Here's how the part is built. I have some questions about the finished solid (model axes, mm). Face numbers are marked on the shaded views. A direction names the side the tool comes from. Round coordinates to 2 decimals unless told otherwise and drop trailing zeros. Write each loop counter-clockwise with the first axis right and the second up, starting at its lowest first coordinate (ties: lowest second). Pieces come first, ordered by that corner, then holes. Notation, with made-up numbers: (-1, -21) - (22, -21) arc R37 cw to (22, 15) - close; hole circle Ø8 at (2, -17). An arc over 180 degrees is marked (long way). Use one line per item in the form item = value. Start each with the question number.
1. Will these pins go through, and if not, where does the flat tip stop? pin 1 (2 mm diameter, centred on x = 65, y = -36, fed in from +Z); pin 2 (10 mm diameter, centred on x = 101.5, z = -59.5, fed in from +Y); pin 3 (1 mm diameter, centred on y = -36, z = -41.5, fed in from +X); pin 4 (3 mm diameter, centred on x = 8.982, z = -11.956, fed in from +Y).
2. I want a section at A-A, the plane x = 96.5. List the corners of the cut face in (y, z) for me, plus the area to 3 significant figures.
3. I want a section at B-B, the plane z = -51.5. List the corners of the cut face in (x, y) for me.
4. Which directions (+Z, -Z, +X, -X, +Y, -Y) give clear straight access to the entire face, cutting with the end or side of a thin tool? Please do the marked faces 1 and 2.
5. We'd pull the mould along Z, two halves only. Please class the marked faces 3 and 4: +Z half, -Z half, draft (parallel to the pull), parting line (faces both ways), or undercut.
6. If I drill on line 1 along Z through (x, y) = (30.5, -38); line 2 along Z through (x, y) = (94.5, -36.25); line 3 along Z through (x, y) = (9, -37.75), over which ranges is the centre line in solid material (lowest first)?
```python
from build123d import *

# Parameters (mm, degrees)
P_IDAT_VYSUNUT_M1_DEPTH      = 2.5
SKICA2_W                     = 43.3
SKICA2_H                     = 10.4
SKICA2_W_2                   = 10.4
SKICA2_H_2                   = 43.3
ODEBRAT_VYSUNUT_M1_DEPTH     = 139.549375892
SKICA6_W                     = 120
SKICA6_H                     = 6.95
P_IDAT_VYSUNUT_M3_DEPTH      = 2
SKICA7_W                     = 5.554617132
SKICA7_H                     = 57.2
SKICA7_W_2                   = 6.443355873
P_IDAT_VYSUNUT_M4_DEPTH      = 2
SKICA3_R                     = 3
P_IDAT_VYSUNUT_M2_DEPTH      = 4
F_2_2_2_2_PR_M_R_D_RY1_D     = 2.2
F_2_2_2_2_PR_M_R_D_RY1_DEPTH = 10
ZAOBLIT1_R                   = 1
SKICA8_W                     = 2.8
SKICA8_H                     = 57.2
ODEBRAT_VYSUNUT_M3_DEPTH     = 139.58455752
F_3_5_3_5_PR_M_R_D_RY1_D     = 3.5
F_3_5_3_5_PR_M_R_D_RY1_DEPTH = 10


with BuildPart() as part:
    # Skica1 → Přidat vysunutím1 (new body)
    with BuildSketch(Plane.XZ.offset(39.4)):
        with BuildLine():
            Line((-4.318, -71.206), (-4.318, -3.206))
            ThreePointArc((-4.318, -3.206), (-2.853533906, 0.329533906), (0.682, 1.794))
            Line((0.682, 1.794), (110.682, 1.794))
            ThreePointArc((110.682, 1.794), (114.217533906, 0.329533906), (115.682, -3.206))
            Line((115.682, -3.206), (115.682, -71.206))
            ThreePointArc((115.682, -71.206), (114.217533906, -74.741533906), (110.682, -76.206))
            Line((110.682, -76.206), (0.682, -76.206))
            ThreePointArc((0.682, -76.206), (-2.853533906, -74.741533906), (-4.318, -71.206))
        make_face()
    extrude(amount=-P_IDAT_VYSUNUT_M1_DEPTH)

    # Skica2 → Odebrat vysunutím1 (cut, through all)
    with BuildSketch(Plane(origin=(0, -36.9, 0), x_dir=(1, 0, 0), z_dir=(0, 1, 0))):
        with Locations((55.682, 3.406)):
            Rectangle(SKICA2_W, SKICA2_H)
        with Locations((0.882, 37.206)):
            Rectangle(SKICA2_W_2, SKICA2_H_2)
        with Locations((55.682, 71.006)):
            Rectangle(SKICA2_W, SKICA2_H)
    extrude(amount=-ODEBRAT_VYSUNUT_M1_DEPTH, mode=Mode.SUBTRACT)

    # Skica6 → Přidat vysunutím3 (add)
    with BuildSketch(Plane(origin=(0, -36.9, 0), x_dir=(1, 0, 0), z_dir=(0, 1, 0))):
        with Locations((55.682, 12.081)):
            Rectangle(SKICA6_W, SKICA6_H)
        with Locations((55.682, 62.331)):
            Rectangle(SKICA6_W, SKICA6_H)
    extrude(amount=P_IDAT_VYSUNUT_M3_DEPTH)

    # Skica7 → Přidat vysunutím4 (add)
    with BuildSketch(Plane(origin=(0, -36.9, 0), x_dir=(1, 0, 0), z_dir=(0, 1, 0))):
        with Locations((105.633212162, 37.206)):
            Rectangle(SKICA7_W, SKICA7_H)
        with Locations((11.204720922, 37.206)):
            Rectangle(SKICA7_W_2, SKICA7_H)
    extrude(amount=P_IDAT_VYSUNUT_M4_DEPTH)

    # Skica3 → Přidat vysunutím2 (add)
    with BuildSketch(Plane(origin=(0, -36.9, 0), x_dir=(1, 0, 0), z_dir=(0, 1, 0))):
        with Locations(Location((30.432, 11.506, 0), (0, 0, 255.164888418))):
            Circle(SKICA3_R)
        with Locations(Location((8.982, 11.956, 0), (0, 0, 270))):
            Circle(SKICA3_R)
        with Locations(Location((8.982, 62.456, 0), (0, 0, 270))):
            Circle(SKICA3_R)
        with Locations(Location((30.432, 62.906, 0), (0, 0, 104.835111582))):
            Circle(SKICA3_R)
        with Locations(Location((80.932, 62.906, 0), (0, 0, 75.164888418))):
            Circle(SKICA3_R)
        with Locations(Location((80.932, 11.506, 0), (0, 0, 284.835111582))):
            Circle(SKICA3_R)
    extrude(amount=P_IDAT_VYSUNUT_M2_DEPTH)

    # Ø2.2 (2.2) průměr díry1
    with Locations(Plane(origin=(0, -39.4, 0), x_dir=(-1, 0, 0), z_dir=(0, -1, 0))):
        with Locations((-8.982, 62.456), (-30.432, 62.906), (-80.932, 62.906), (-80.932, 11.506), (-30.432, 11.506), (-8.982, 11.956)):
            Hole(F_2_2_2_2_PR_M_R_D_RY1_D / 2, depth=F_2_2_2_2_PR_M_R_D_RY1_DEPTH)

    # Zaoblit1
    zaoblit1_edges = [part.edges().sort_by_distance(p)[0] for p in [
        (80.932, -36.9, -8.506),
        (80.932, -36.9, -65.906),
        (30.432, -36.9, -65.906),
    ]]
    fillet(zaoblit1_edges, radius=ZAOBLIT1_R)

    # Skica8 → Odebrat vysunutím3 (cut, through all)
    with BuildSketch(Plane(origin=(0, -36.9, 0), x_dir=(1, 0, 0), z_dir=(0, 1, 0))):
        with Locations((-2.918, 37.206)):
            Rectangle(SKICA8_W, SKICA8_H)
        with Locations((114.282, 37.206)):
            Rectangle(SKICA8_W, SKICA8_H)
    extrude(amount=ODEBRAT_VYSUNUT_M3_DEPTH, mode=Mode.SUBTRACT)

    # Ø3.5 (3.5) průměr díry1
    with Locations(Plane(origin=(0, -39.4, 0), x_dir=(-1, 0, 0), z_dir=(0, -1, 0))):
        with Locations((0, 2.696455625), (-0.682, 71.206), (-110.682, 71.206), (-110.682, 3.206)):
            Hole(F_3_5_3_5_PR_M_R_D_RY1_D / 2, depth=F_3_5_3_5_PR_M_R_D_RY1_DEPTH)


solid = part.part
```
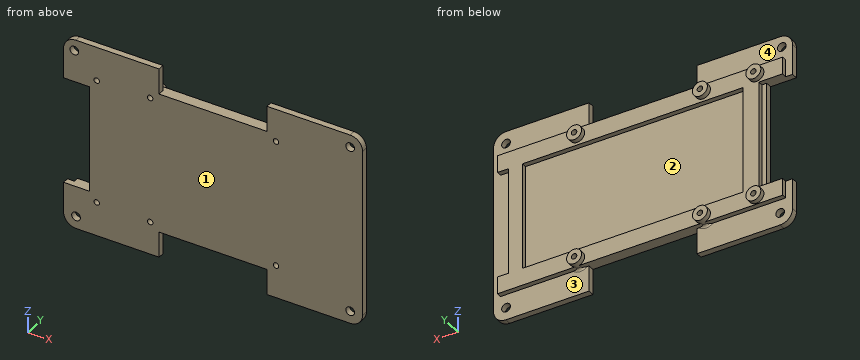
Model answer:
q1.pin_1 = -8.61
q1.pin_2 = -34.9
q1.pin_3 = 108.41
q1.pin_4 = -32.9
q2.outline = (-39.4, -76.21) - (-36.9, -76.21) - (-36.9, -65.81) - (-34.9, -65.81) - (-34.9, -58.86) - (-36.9, -58.86) - (-36.9, -15.56) - (-34.9, -15.56) - (-34.9, -8.61) - (-36.9, -8.61) - (-36.9, 1.79) - (-39.4, 1.79) - close
q2.area = 223 mm2
q3.outline = (6.08, -39.4) - (115.68, -39.4) - (115.68, -36.9) - (108.41, -36.9) - (108.41, -34.9) - (102.86, -34.9) - (102.86, -36.9) - (14.43, -36.9) - (14.43, -34.9) - (7.98, -34.9) - (7.98, -36.9) - (6.08, -36.9) - close
q4.face_1 = +Z, -Z, +X, -X, -Y
q4.face_2 = +Y
q5.face_3 = undercut
q5.face_4 = draft
q6.line_1 = -76.21 to -64, -61.81 to -12.6, -10.41 to 1.79
q6.line_2 = -65.81 to -58.86, -15.56 to -8.61
q6.line_3 = -76.21 to -63.56, -61.36 to -13.06, -10.86 to 1.79
